from build123d import *

# Parameters (mm, degrees)
MODEL_R             = 3.6
MODEL_R_2           = 0.75
MODEL_R_3           = 1.500000002
MODEL_R_4           = 1.3
MODEL_R_5           = 1.5
BOSS_EXTRUDE1_DEPTH = 3


with BuildPart() as part:
    # Model → Boss-Extrude1 (new body)
    with BuildSketch(Plane.XY):
        with BuildLine():
            Line((43.808, 64.448), (43.808, 61.448))
            Line((43.808, 61.448), (36.308, 61.448))
            Line((36.308, 61.448), (36.308, 70.448))
            Line((36.308, 70.448), (-22.414233443, 70.448))
            ThreePointArc((-22.414233443, 70.448), (-26.027950405, 69.188749962), (-27.692809934, 65.743041952))
            Line((-27.692809934, 65.743041952), (-27.692809934, 14.360233482))
            ThreePointArc((-27.692809934, 14.360233482), (-26.128440702, 10.72754285), (-22.414233443, 9.368))
            Line((-22.414233443, 9.368), (36.308, 9.368))
            Line((36.308, 9.368), (36.308, 18.368))
            Line((36.308, 18.368), (43.808, 18.368))
            Line((43.808, 18.368), (43.808, 15.368))
            Line((43.808, 15.368), (53.808, 15.368))
            Line((53.808, 15.368), (53.808, 18.368))
            Line((53.808, 18.368), (64.808, 18.368))
            Line((64.808, 18.368), (64.808, 22.368))
            Line((64.808, 22.368), (63.508, 22.368))
            Line((63.508, 22.368), (63.508, 24.868))
            Line((63.508, 24.868), (64.808, 24.868))
            Line((64.808, 24.868), (64.808, 26.368))
            Line((64.808, 26.368), (67.808, 26.368))
            Line((67.808, 26.368), (67.808, 24.868))
            Line((67.808, 24.868), (69.108, 24.868))
            Line((69.108, 24.868), (69.108, 22.368))
            Line((69.108, 22.368), (67.808, 22.368))
            Line((67.808, 22.368), (67.808, 18.368))
            Line((67.808, 18.368), (78.808, 18.368))
            Line((78.808, 18.368), (78.808, 15.368))
            Line((78.808, 15.368), (88.808, 15.368))
            Line((88.808, 15.368), (88.808, 18.368))
            Line((88.808, 18.368), (90.308, 18.368))
            Line((90.308, 18.368), (90.308, 61.448))
            Line((90.308, 61.448), (88.808, 61.448))
            Line((88.808, 61.448), (88.808, 64.448))
            Line((88.808, 64.448), (78.808, 64.448))
            Line((78.808, 64.448), (78.808, 61.448))
            Line((78.808, 61.448), (67.808, 61.448))
            Line((67.808, 61.448), (67.808, 57.4481))
            Line((67.808, 57.4481), (69.108, 57.4481))
            Line((69.108, 57.4481), (69.108, 54.9481))
            Line((69.108, 54.9481), (67.808, 54.9481))
            Line((67.808, 54.9481), (67.808, 53.448))
            Line((67.808, 53.448), (64.808, 53.448))
            Line((64.808, 53.448), (64.808, 54.9481))
            Line((64.808, 54.9481), (63.508, 54.9481))
            Line((63.508, 54.9481), (63.508, 57.4481))
            Line((63.508, 57.4481), (64.808, 57.4481))
            Line((64.808, 57.4481), (64.808, 61.448))
            Line((64.808, 61.448), (53.808, 61.448))
            Line((53.808, 61.448), (53.808, 64.448))
            Line((53.808, 64.448), (43.808, 64.448))
        make_face()
        with Locations((66.20800481, 39.598049108)):
            Circle(MODEL_R, mode=Mode.SUBTRACT)
        with Locations((55.207943868, 39.587694441)):
            Circle(MODEL_R_2, mode=Mode.SUBTRACT)
        with Locations((66.20800481, 46.298)):
            Circle(MODEL_R_2, mode=Mode.SUBTRACT)
        with Locations((66.20800481, 32.898)):
            Circle(MODEL_R_2, mode=Mode.SUBTRACT)
        with Locations((77.20800481, 39.598049108)):
            Circle(MODEL_R_2, mode=Mode.SUBTRACT)
        with Locations((85.058, 48.068)):
            Circle(MODEL_R_3, mode=Mode.SUBTRACT)
        with Locations((30.908, 41.668)):
            Circle(MODEL_R_4, mode=Mode.SUBTRACT)
        with Locations((86.808, 41.668)):
            Circle(MODEL_R_4, mode=Mode.SUBTRACT)
        with Locations((30.908, 22.868)):
            Circle(MODEL_R_4, mode=Mode.SUBTRACT)
        with Locations((86.808, 22.868)):
            Circle(MODEL_R_4, mode=Mode.SUBTRACT)
        with Locations((1.635766557, 67.408)):
            Circle(MODEL_R_5, mode=Mode.SUBTRACT)
        with Locations((24.635766557, 67.408)):
            Circle(MODEL_R_5, mode=Mode.SUBTRACT)
        with Locations((1.635766557, 12.408)):
            Circle(MODEL_R_5, mode=Mode.SUBTRACT)
        with Locations((24.635766557, 12.408)):
            Circle(MODEL_R_5, mode=Mode.SUBTRACT)
    extrude(amount=BOSS_EXTRUDE1_DEPTH)


solid = part.part
Can you work these out from the model? Positions are in its coordinate system, mm. A direction names the side the tool comes from. Give positions to 0.01 mm unless a question says otherwise; leave off trailing zeros. One line per item, written item: value. Start each with the question number.
1) Thinking about a two-plate mould opening in Y: for faces 4 (the face through (78.808, 63, 1)), 5 (the face through (26.02, 66.83, 1.48)), 6 (the face through (73, 61.448, 1)), which applies, +Y half, -Y half, draft (parallel to the pull), parting line (faces both ways), or undercut?
2) If I drill on line 1 (X direction, y = 61.5, z = 1.2); line 2 (X direction, y = 61, z = 1.6); line 3 (X direction, y = 55.5, z = 1.5), over which ranges is the centre line in solid material (lowest first)? Write a range as [from, to].
3) If we section it at A-A, the plane z = 1.1: Give the number of separate pieces and of enclosed holes in the cut face, and give its area (3 significant figures).
4) On a 3-axis mill with a long thin cutter (end or side, diameter ignored), from which of +Z, -Z, +X, -X, +Y, -Y can I reach the whole of each face in a straight line? I mean faces 1 (the face through (64.808, 20, 1)), 2 (the face through (49, 64.448, 1)), 3 (the face through (36.308, 66, 1)). Say none if no direction works.
5) I'm going to push flat-ended pins straight in: pin 1 (0.8 mm diameter, centred on x = 89, z = 1.5, fed in from +Y); pin 2 (2.5 mm diameter, centred on x = 1.64, y = 67.41, fed in from -Z); pin 3 (1.5 mm diameter, centred on x = 72.5, z = 2, fed in from +Y). Where does each tip first touch, or does it pass through?
Completed:
1. face 4: draft
1. face 5: undercut
1. face 6: +Y half
2. line 1: x = [-27.69, 36.31], [43.81, 53.81], [78.81, 88.81]
2. line 2: x = [-27.69, 64.81], [67.81, 90.31]
2. line 3: x = [-27.69, 63.51], [69.11, 90.31]
3. separate pieces: 1
3. enclosed holes: 14
3. area: 6,180 mm^2
4. face 1: +Z, -Z, -Y
4. face 2: +Z, -Z, +X, +Y
4. face 3: +Z, -Z, +Y
5. pin 1: stops at y = 64.45
5. pin 2: passes through
5. pin 3: stops at y = 61.45
